Source: CAD feature listing. Evaluate the final solid. Frame: model axes, mm. Give positions to 0.01 mm unless a question says otherwise; leave off trailing zeros. Loops run counter-clockwise (first coordinate to the right, second up) from the corner with the lowest first, then second, coordinate; pieces in that order, holes last. Notation, with made-up numbers: M 11.25,-21 L 50.25,-21 A25 cw 50.25,9 Z; hole C 57.25,48.25 d4. An arc over 180 degrees is marked long. Answer in a Markdown table with one row per item.
```python
from build123d import *

# Parameters (mm, degrees)
CONG_1_R       = 1.1
ECHELLE1_SCALE = 0.69


with BuildPart() as part:
    # Esquisse2 → Révolution1 (revolve)
    with BuildSketch(Plane(origin=(0, 0, 0), x_dir=(0, 0, -1), z_dir=(1, 0, 0)), mode=Mode.PRIVATE) as r_volution1_sk:
        with BuildLine():
            Line((-7.5, 14.8), (-7.5, 10))
            Line((-7.5, 10), (7.5, 10))
            Line((7.5, 10), (7.5, 14.8))
            Line((7.5, 14.8), (3.577708764, 14.8))
            ThreePointArc((3.577708764, 14.8), (0, 13.2), (-3.577708764, 14.8))
            Line((-3.577708764, 14.8), (-7.5, 14.8))
        make_face()
    revolve(r_volution1_sk.sketch.rotate(Axis((0, 0, 0), (0, 0, 1)), 90), axis=Axis((0, 0, 0), (0, 0, 1)))

    # Congé1
    cong_1_edges = [part.edges().sort_by_distance(p)[0] for p in [
        (10, 0, -7.5),
        (10, 0, 7.5),
    ]]
    fillet(cong_1_edges, radius=CONG_1_R)


with BuildPart() as part_1:
    # Echelle1: scaled about (0, 0, 0)
    add(part.part.scale(ECHELLE1_SCALE))


solid = part_1.part
```
1) Material intervals for L1, parallel to Y at x = 0, z = 2.5; L2, parallel to X at y = 5, z = -3 (3 decimals); L3, parallel to Y at x = 3, z = -3, sorted ascending.
Reply:
| item | result |
|---|---|
| L1 | y = -10.21 to -6.9, 6.9 to 10.21 |
| L2 | x = -8.904 to -4.755, 4.755 to 8.904 |
| L3 | y = -9.76 to -6.21, 6.21 to 9.76 |
2) Pull-direction query (X, two-part tool) for faces 1 (the flat face through (1, -8, -5.175)), 2 (the cylindrical face through (5.09, -4.66, -0.06)), 3 (the cylindrical face through (-4.71, 9.06, 3.84)); classes: released by +X, released by -X, zero draft, split by the parting line, or undercut.
Reply:
| item | result |
|---|---|
| face 1 | zero draft |
| face 2 | undercut |
| face 3 | split by the parting line |
3) Section A-A, the plane x = 0. Return loops of the section in (y, z) (3 decimals), then the cut area to 3 significant figures.
Reply:
| item | result |
|---|---|
| outline | M -10.212,-5.175 L -7.659,-5.175 A0.759 ccw -6.9,-4.416 L -6.9,4.416 A0.759 ccw -7.659,5.175 L -10.212,5.175 L -10.212,2.469 A3.312 cw -10.212,-2.469 Z; M 6.9,-4.416 A0.759 ccw 7.659,-5.175 L 10.212,-5.175 L 10.212,-2.469 A3.312 cw 10.212,2.469 L 10.212,5.175 L 7.659,5.175 A0.759 ccw 6.9,4.416 Z |
| area | 60.5 mm² |
4) Section C-C, the plane z = 4. Return loops of the section in (x, y), then the cut area to 3 significant figures.
Reply:
| item | result |
|---|---|
| outline | C 0,0 d20.42; hole C 0,0 d13.8 |
| area | 178 mm² |
5) Pin query (flat end, axial travel): pin 1 Ø1.5 at (x, z) = (5.5, 3) entering from +Y; pin 2 Ø5 at (y, z) = (-4, 2) entering from -X; pin 3 Ø1.5 at (x, z) = (1, -0.5) entering from +Y. Return the tip coordinate at first contact, or that it passes through.
Reply:
| item | result |
|---|---|
| pin 1 | stops at y = 9.04 |
| pin 2 | stops at x = -10.09 |
| pin 3 | stops at y = 9.31 |
6) Section D-D, the plane z = -1.75. Return loops of the section in (x, y).
Reply:
| item | result |
|---|---|
| outline | C 0,0 d19.22; hole C 0,0 d13.8 |
